Autodesk Inventor part; units mm, degrees
ref_plane "YZ Plane" through (0, 0, 0) normal (1, 0, 0) x (0, 1, 0)
ref_plane "XZ Plane" through (0, 0, 0) normal (0, 1, 0) x (-1, 0, 0)
ref_plane "XY Plane" through (0, 0, 0) normal (0, 0, 1) x (1, 0, 0)
sketch "Sketch1" plane through (0, 0, 0) normal (0, 1, 0) x (-1, 0, 0)
  circle A0 centre (0, 0) radius 39.5
  circle A1 centre (0, 0) radius 36.5
  circle A2 centre (0, 45) radius 3.5
  circle A3 centre (0, 45) radius 2
  arc A4 (3.02, 46.7691) -> (14.7602, 36.6386) centre (23.7285, 58.9) ccw
  arc A5 (-14.7602, 36.6386) -> (-3.02, 46.7691) centre (-23.7285, 58.9) ccw
  arc A6 (-46.7691, 3.02) -> (-36.6386, 14.7602) centre (-58.9, 23.7285) ccw
  circle A7 centre (-45, 0) radius 3.5
  circle A8 centre (-45, 0) radius 2
  arc A9 (-36.6386, -14.7602) -> (-46.7691, -3.02) centre (-58.9, -23.7285) ccw
  arc A10 (-3.02, -46.7691) -> (-14.7602, -36.6386) centre (-23.7285, -58.9) ccw
  circle A11 centre (0, -45) radius 3.5
  circle A12 centre (0, -45) radius 2
  arc A13 (14.7602, -36.6386) -> (3.02, -46.7691) centre (23.7285, -58.9) ccw
  arc A14 (46.7691, -3.02) -> (36.6386, -14.7602) centre (58.9, -23.7285) ccw
  circle A15 centre (45, 0) radius 3.5
  circle A16 centre (45, 0) radius 2
  arc A17 (36.6386, 14.7602) -> (46.7691, 3.02) centre (58.9, 23.7285) ccw
  point P0 (36.6386, 14.7602)
  point P1 (-36.6386, 14.7602)
  point P2 (-36.6386, -14.7602)
  point P3 (-14.7602, -36.6386)
  point P4 (14.7602, -36.6386)
  point P5 (36.6386, -14.7602)
  dimension "d0" = 79
  dimension "d1" = 73
  dimension "d2" = 7
  dimension "d3" = 4
  dimension "d8" = 360
  dimension "d12" = 45
  dimension "d13" = 24
extrude "Extrusion1" add sketch "Sketch1" along normal blind 5 contours A0 | A0 A17 A15 A14 | A0 A5 A2 A4 | A15 | A13 A11 A10 A0 | A2 | A11 | A0 A9 A7 A6 | A7 | A1
properties part number "tapa"
Design review of the part built by this model. Coordinates are the model's own, in mm. Round coordinates to 2 decimals unless told otherwise and drop trailing zeros. Write each loop counter-clockwise with the first axis right and the second up, starting at its lowest first coordinate (ties: lowest second). Pieces come first, ordered by that corner, then holes.
Item 1: We need section C-C on z = -45. Write out the cut boundary in (x, y).
Item 2: The part is to be moulded in two halves that separate along Z. For faces 1 (the cylindrical face through (-40.66, 2.46, -8.13)), 2 (the cylindrical face through (0, 2, 47)), 3 (the cylindrical face through (-48.5, 2.5, 0.1)), say which applies: +Z half, -Z half, draft (parallel to the pull), parting line (faces both ways), or undercut.
Item 3: Clearance check with flat-ended pins moving along their axes: pin 1 Ø4.5 at (x, z) = (-45, 0) entering from +Y; pin 2 Ø2 at (x, y) = (16, 4.5) entering from -Z. State where each tip first meets the part, or that it passes through.
Item 4: For probe 1 along Z at (x, y) = (-45, 3.8); probe 2 along X at (y, z) = (0.95, -11.5); probe 3 along Z at (x, y) = (39, 1.8), list the stretches that pass through material, from the lowest coordinate up.
Item 5: We need section D-D on x = -45. Write out the cut boundary in (y, z), and give its area (3 significant figures).
Item 6: We need section B-B on x = 0. Write out the cut boundary in (y, z), and give its area (3 significant figures).
Item 7: We need section A-A on z = 0. Write out the cut boundary in (x, y).
Returned:
1. outline: (-4.16, 0) - (-2, 0) - (-2, 5) - (-4.16, 5) - close; (2, 0) - (4.16, 0) - (4.16, 5) - (2, 5) - close
2. face 1: -Z half
2. face 2: undercut
2. face 3: parting line
3. pin 1: stops at y = 5
3. pin 2: stops at z = -36.54
4. probe 1: z = -4.16 to -2, 2 to 4.16
4. probe 2: x = -38.25 to 38.25
4. probe 3: z = -10.31 to 10.31
5. outline: (0, -4.16) - (5, -4.16) - (5, -2) - (0, -2) - close; (0, 2) - (5, 2) - (5, 4.16) - (0, 4.16) - close
5. area: 21.6 mm2
6. outline: (0, -48.5) - (5, -48.5) - (5, -47) - (0, -47) - close; (0, -43) - (5, -43) - (5, 43) - (0, 43) - close; (0, 47) - (5, 47) - (5, 48.5) - (0, 48.5) - close
6. area: 445 mm2
7. outline: (-48.5, 0) - (-47, 0) - (-47, 5) - (-48.5, 5) - close; (-43, 0) - (43, 0) - (43, 5) - (-43, 5) - close; (47, 0) - (48.5, 0) - (48.5, 5) - (47, 5) - close
